Work out the finished part from the listing and answer in its coordinate system (mm). Round coordinates to 2 decimals unless told otherwise and drop trailing zeros. Loops run counter-clockwise (first coordinate to the right, second up) from the corner with the lowest first, then second, coordinate; pieces in that order, holes last. Notation, with made-up numbers: (-1, -28.75) -> (36, -28.75) arc R23 ccw to (36, -14.75) -> close; hole circle Ø3 at (52.5, 82). An arc over 180 degrees is marked (long way). Write item = value, one per line. Start each with the question number.
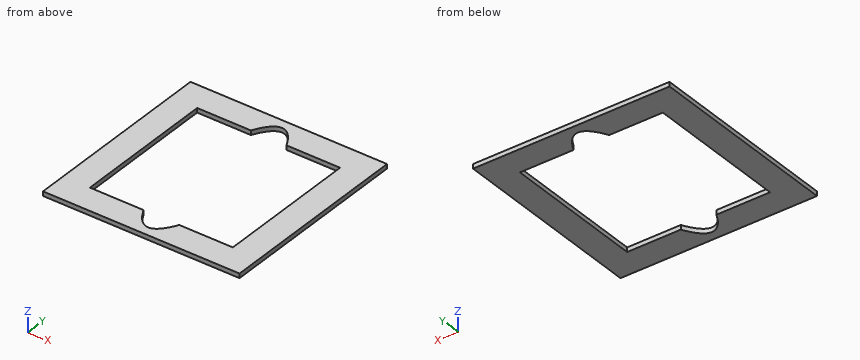
```python
from build123d import *

# Parameters (mm, degrees)
SKETCH1_W           = 139.7
SKETCH1_H           = 139.7
BOSS_EXTRUDE1_DEPTH = 3.175


with BuildPart() as part:
    # Sketch1 → Boss-Extrude1 (new body)
    with BuildSketch(Plane.XY):
        with Locations((69.85, 69.85)):
            Rectangle(SKETCH1_W, SKETCH1_H)
        with BuildLine():
            Line((19.05, 120.65), (57.15, 120.65))
            add(Edge.make_bspline(
                [(57.15, 120.65), (69.85, 146.05), (82.55, 120.65)],
                knots=[0, 0, 0, 1, 1, 1], degree=2))
            Line((82.55, 120.65), (120.65, 120.65))
            Line((120.65, 120.65), (120.65, 19.05))
            Line((120.65, 19.05), (82.55, 19.05))
            add(Edge.make_bspline(
                [(57.15, 19.05), (69.85, -6.155350719), (82.55, 19.05)],
                knots=[0, 0, 0, 1, 1, 1], degree=2))
            Line((57.15, 19.05), (19.05, 19.05))
            Line((19.05, 19.05), (19.05, 120.65))
        make_face(mode=Mode.SUBTRACT)
    extrude(amount=BOSS_EXTRUDE1_DEPTH)


solid = part.part
```
Item 1: Section A-A (x = 105.5) is taken. Determine the outline of the cut face in (y, z) (3 decimals), then the cut area to 3 significant figures.
Item 2: Find the intervals of material crossed by line 1 along X through (y, z) = (56.5, 1.3); line 2 along Y through (x, z) = (69.5, 1.05), in increasing order. Write a range as [from, to].
Item 3: A flat-ended cylindrical pin translates along its axis: pin 1 (1.6 mm diameter, centred on y = 64, z = 1.5, fed in from -X). Find the tip coordinate at first contact, or state that the pin passes through.
Worked answers:
q1.outline = (0, 0) -> (19.05, 0) -> (19.05, 3.175) -> (0, 3.175) -> close; (120.65, 0) -> (139.7, 0) -> (139.7, 3.175) -> (120.65, 3.175) -> close
q1.area = 121 mm2
q2.line_1 = [0, 19.05], [120.65, 139.7]
q2.line_2 = [0, 6.46], [133.34, 139.7]
q3.pin_1 = 0
